Design review of the part built by this model. Coordinates are the model's own, in mm. Face numbers are marked on the shaded views. A direction names the side the tool comes from. Give positions to 0.01 mm unless a question says otherwise; leave off trailing zeros. Order: outer loops, then holes, each group sorted by start corner. A loop starts at its lowest first (then second) coordinate and runs counter-clockwise, first axis right, second up. Notation, with made-up numbers: M 7,-25 L 52,-25 A23 ccw 52,-16 Z; hole C -30.75,22.5 d9. An arc over 180 degrees is marked long. Answer as a JSON object with one key per item and string values.
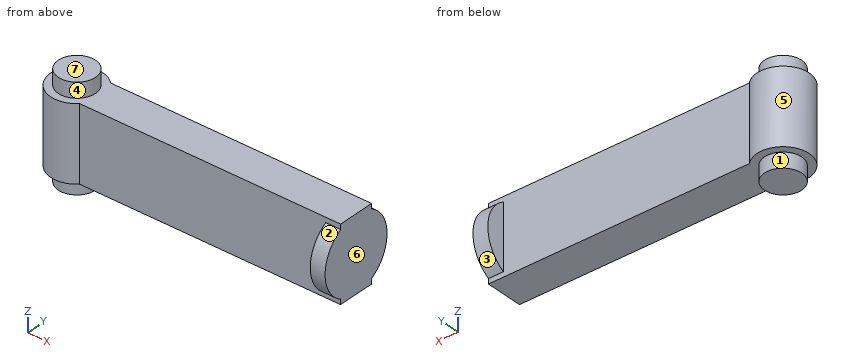
from build123d import *

# Parameters (mm, degrees)
BOSS_EXTRUDE1_DEPTH      = 100
SKETCH2_R                = 50
BOSS_EXTRUDE2_DEPTH      = 20
SKETCH3_R                = 25
BOSS_EXTRUDE3_DEPTH      = 20
BOSS_EXTRUDE3_DEPTH_BACK = 120


with BuildPart() as part:
    # Sketch1 → Boss-Extrude1 (new body)
    with BuildSketch(Plane.XY):
        with BuildLine():
            Line((24.494897428, 25), (375, 25))
            Line((375, 25), (375, -25))
            Line((375, -25), (24.494897428, -25))
            ThreePointArc((24.494897428, -25), (-35, 0), (24.494897428, 25))
        make_face()
    extrude(amount=BOSS_EXTRUDE1_DEPTH)

    # Sketch2 → Boss-Extrude2 (add)
    with BuildSketch(Plane(origin=(375, 0, 0), x_dir=(0, 0, -1), z_dir=(1, 0, 0))):
        with Locations((-50, 0)):
            Circle(SKETCH2_R)
    extrude(amount=-BOSS_EXTRUDE2_DEPTH)

    # Sketch3 → Boss-Extrude3 (add, two sides)
    with BuildSketch(Plane.XY.offset(100)) as boss_extrude3_sk:
        Circle(SKETCH3_R)
    extrude(amount=BOSS_EXTRUDE3_DEPTH)
    extrude(boss_extrude3_sk.sketch, amount=-BOSS_EXTRUDE3_DEPTH_BACK)


solid = part.part
(1) We need section A-A (x = 0). Write out the cut boundary in (y, z).
Checked values:
{"outline": "M -35,0 L -25,0 L -25,-20 L 25,-20 L 25,0 L 35,0 L 35,100 L 25,100 L 25,120 L -25,120 L -25,100 L -35,100 Z"}
(2) We need section B-B (z = 21.5). Write out the cut boundary in (x, y), plus the area to 3 significant figures.
Checked values:
{"outline": "M 24.49,-25 L 355,-25 L 355,-41.08 L 375,-41.08 L 375,41.08 L 355,41.08 L 355,25 L 24.49,25 A35 ccw long Z", "area": "21,700 mm^2"}
(3) We need section D-D (z = 57). Write out the cut boundary in (x, y).
Checked values:
{"outline": "M 24.49,-25 L 355,-25 L 355,-49.51 L 375,-49.51 L 375,49.51 L 355,49.51 L 355,25 L 24.49,25 A35 ccw long Z"}
(4) Insertion check: pin 1 (8 mm diameter, centred on x = 330, y = -12, fed in from +Z); pin 2 (4 mm diameter, centred on x = 93.5, z = 62.5, fed in from -Y); pin 3 (21 mm diameter, centred on x = 268, y = 11, fed in from -Z); pin 4 (12 mm diameter, centred on x = 199, y = 36.5, fed in from +Z). Each pin has a flat end and moves straight along its axis. Give the tip position at first contact, or say it passes through.
Checked values:
{"pin 1": "stops at z = 100", "pin 2": "stops at y = -25", "pin 3": "stops at z = 0", "pin 4": "passes through"}
(5) Tool access review of the marked faces 1, 2 and 3: name each direction out of +Z, -Z, +X, -X, +Y, -Y from which nothing blocks a thin tool from reaching the whole face with its end or side.
Checked values:
{"face 1": "-Z", "face 2": "+X, -Y", "face 3": "+X, +Y"}
(6) To check wall thickness, follow L1, parallel to Y at x = 130.5, z = 7; L2, parallel to Z at x = 110.5, y = -5.5; L3, parallel to X at y = 17, z = 79. State the ranges of each line that lie inside material, in increasing order. Write a range as from..to.
Checked values:
{"L1": "y = -25..25", "L2": "z = 0..100", "L3": "x = -30.59..375"}
(7) We need section C-C (y = 0). Write out the cut boundary in (x, z).
Checked values:
{"outline": "M -35,0 L -25,0 L -25,-20 L 25,-20 L 25,0 L 375,0 L 375,100 L 25,100 L 25,120 L -25,120 L -25,100 L -35,100 Z"}
(8) Draft analysis for pull direction X (two halves, no side actions). For the marked faces 4, 5, 6 and 7, state which applies: +X half, -X half, draft (parallel to the pull), parting line (faces both ways), or undercut.
Checked values:
{"face 4": "parting line", "face 5": "undercut", "face 6": "+X half", "face 7": "draft"}
